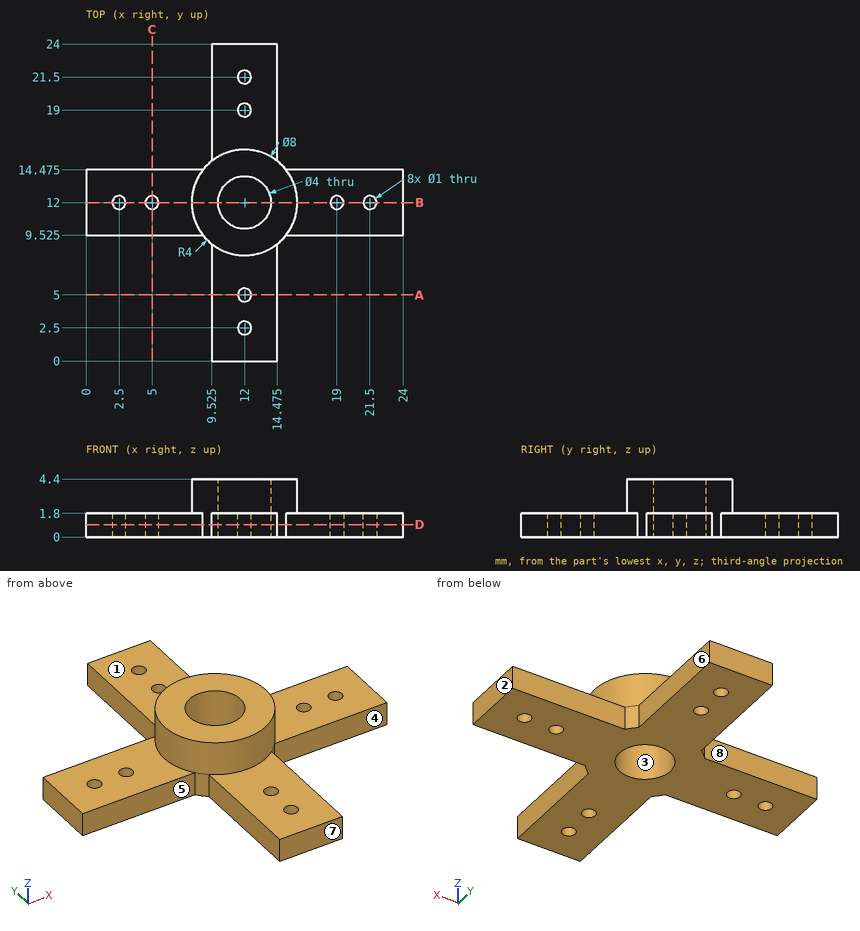
Answer from the drawing. Dimensions are ordinates in mm from the lowest x, y and z of the part. A direction names the side the tool comes from. Round coordinates to 2 decimals unless told otherwise and drop trailing zeros. Write each loop counter-clockwise with the first axis right and the second up, starting at its lowest first coordinate (ties: lowest second). Pieces come first, ordered by that corner, then holes. Notation, with made-up numbers: (-33.75, 3) - (-26.75, 3) arc R14 cw to (-26.75, 24) - close; hole circle Ø7 at (9.5, 32.5). An arc over 180 degrees is marked (long way). One line per item, written item: value.
Q1. Find section A-A (y = 5). Determine the outline of the cut face in (x, z) (3 decimals).
The answers:
outline: (9.525, 0) - (11.5, 0) - (11.5, 1.8) - (9.525, 1.8) - close; (12.5, 0) - (14.475, 0) - (14.475, 1.8) - (12.5, 1.8) - close
Q2. Find section D-D (z = 0.95). Count the separate pieces of the cut face and the enclosed holes in it, and give its area (3 significant figures).
The answers:
separate pieces: 1
enclosed holes: 9
area: 195 mm2
Q3. Which of the six approach directions +Z, -Z, +X, -X, +Y, -Y give full straight-line access (tool end or side, diameter ignored) to the marked faces 4, 5, 6, 7 and 8?
The answers:
face 4: +Z, -Z, +X, -Y
face 5: +Z, -Z, -X, -Y
face 6: +Z, -Z, +X, +Y
face 7: +Z, -Z, +X, -X, -Y
face 8: +Z, -Z, -X, +Y
Q4. For a pull along X with two mould halves and no side action, classify the marked faces 1, 2 and 3 as pulls with the +X half, pulls with the -X half, needs draft (parallel to the pull), parting line crosses it, or undercut.
The answers:
face 1: needs draft
face 2: pulls with the +X half
face 3: undercut
Q5. Straight lines are drawn through the part: line 1 (Y direction, x = 12, z = 1.1); line 2 (X direction, y = 5, z = 1.2) (3 decimals). For each, find the intervals that lie inside material, in ascending order. Write a range as from..to.
The answers:
line 1: y = 0..2, 3..4.5, 5.5..10, 14..18.5, 19.5..21, 22..24
line 2: x = 9.525..11.5, 12.5..14.475
Q6. Each of these flat-tipped pins is pushed along its axis until it touches: P1, Ø0.5, axis at y = 18.5, z = 1, coming from the +X side (3 decimals); P2, Ø0.9, axis at x = 21, z = 0.5, coming from the +Y side (3 decimals); P3, Ø5.5, axis at x = 12.5, y = 3, coming from the +Z side; P4, Ø4, axis at x = 20.5, y = 7, coming from the +Z side. Where does it stop, or does it pass through?
The answers:
P1: stops at x = 14.475
P2: stops at y = 14.475
P3: stops at z = 1.8
P4: passes through
Q7. Find section B-B (y = 12). Determine the outline of the cut face in (x, z).
The answers:
outline: (0, 0) - (2, 0) - (2, 1.8) - (0, 1.8) - close; (3, 0) - (4.5, 0) - (4.5, 1.8) - (3, 1.8) - close; (5.5, 0) - (10, 0) - (10, 4.4) - (8, 4.4) - (8, 1.8) - (5.5, 1.8) - close; (14, 0) - (18.5, 0) - (18.5, 1.8) - (16, 1.8) - (16, 4.4) - (14, 4.4) - close; (19.5, 0) - (21, 0) - (21, 1.8) - (19.5, 1.8) - close; (22, 0) - (24, 0) - (24, 1.8) - (22, 1.8) - close
